```python
from build123d import *

# Parameters (mm, degrees)
F2_R = 5.08
F3_R = 5.08


with BuildPart() as f1:
    # F0 (on Front) → F1 (revolve)
    with BuildSketch(Plane.XZ):
        Polygon((0, -27.148815), (0, 59.899766), (-14.939032, 59.899766), (-14.939032, 48.982784), (-9.767827, 48.982784), (-9.767827, 44.098869), (-15.51361, 39.789535), (-20.397522, 37.203934), (-25.558326, 31.527043), (-20.110233, 26.574237), (-23.844991, 20.541167), (-23.844991, -4.165691), (-23.844991, -27.148815), align=None)
    revolve(axis=Axis((0, 0, 16.375476), (0, 0, 1)))

    # F2
    f2_edges = [f1.edges().sort_by_distance(p)[0] for p in [
        (20.110233, 0, 26.574237),
        (23.844991, 0, 20.541167),
        (-21.977612, 0, 23.557702),
    ]]
    fillet(f2_edges, radius=F2_R)

    # F3
    f3_edges = [f1.edges().sort_by_distance(p)[0] for p in [
        (25.558326, 0, 31.527043),
    ]]
    fillet(f3_edges, radius=F3_R)


solid = f1.part
```
Work out the finished part from the listing and answer in its coordinate system (mm). A direction names the side the tool comes from. Coordinates: 2 decimals unless noted, no trailing zeros. Loops run counter-clockwise (first coordinate to the right, second up) from the corner with the lowest first, then second, coordinate; pieces in that order, holes last. Notation, with made-up numbers: (17.5, -22) -> (52.5, -22) arc R18 cw to (52.5, -8) -> close; hole circle Ø4 at (-12.5, -30). An arc over 180 degrees is marked (long way). Answer as CSV lines item,"result".
Q1. A tool of negligible diameter and unlimited length cuts with its end or side. For faces 4 (the face through (-3, 10, 48.983)), 5 (the face through (0, 0, 59.9)), 6 (the face through (-6.893, 13.253, 54.365)), from which of +Z, -Z, +X, -X, +Y, -Y can it reach the whole face along a straight path? Write none if from no direction.
Findings:
face 4,"none"
face 5,"+Z, +X, -X, +Y, -Y"
face 6,"+Z"
Q2. Each of these flat-tipped pins is pushed along its axis until it touches: pin 1 (2 mm diameter, centred on x = -6.5, y = -14.5, fed in from +Z); pin 2 (12 mm diameter, centred on y = -5.5, z = 41.5, fed in from +X); pin 3 (8 mm diameter, centred on x = 1, z = 39, fed in from -Y); pin 4 (6 mm diameter, centred on x = -8, z = 20.5, fed in from +Y). Where does it stop, or does it pass through?
Findings:
pin 1,"stops at z = 59.9"
pin 2,"stops at x = 21.41"
pin 3,"stops at y = -22.38"
pin 4,"stops at y = 23.26"
Q3. Find the intervals of material crossed by probe 1 along Z at (x, y) = (12, -5); probe 2 along Z at (x, y) = (-8.5, -10); probe 3 along Z at (x, y) = (-20, -1), in increasing order.
Findings:
probe 1,"z = -27.15 to 41.67, 48.98 to 59.9"
probe 2,"z = -27.15 to 41.58, 48.98 to 59.9"
probe 3,"z = -27.15 to 37.4"
Q4. The part is cut by section B-B on z = 5. Write down the section's boundary in (x, y) (3 decimals), and give its area (3 significant figures).
Findings:
outline,"circle Ø47.69 at (0, 0)"
area,"1,790 mm²"
Q5. For a pull along Z with two mould halves and no side action, classify faces 1 (the face through (-15.089, -4.752, 39.628)), 2 (the face through (5.169, 23.278, -4.35)), 3 (the face through (2.195, 9.886, 43.829)) as +Z half, -Z half, draft (parallel to the pull), parting line (faces both ways), or undercut.
Findings:
face 1,"+Z half"
face 2,"draft"
face 3,"undercut"
Q6. The part is cut by section A-A on z = 46.5. Write down the section's boundary in (x, y).
Findings:
outline,"circle Ø19.54 at (0, 0)"
